```python
from build123d import *

# Parameters (mm, degrees)
BOSS_EXTRU_1_DEPTH = 3


with BuildPart() as part:
    # Esquisse1 → Boss.-Extru.1 (new body)
    with BuildSketch(Plane.XY):
        Polygon((-113.35310374, -10.173637327), (-129.143746737, -14.701531345), (-206.446773007, -14.701531345), (-222.237416003, -10.173637327), (-228.962816583, -8.245159743), (-248.413999189, -2.668793647), (-249.872259625, -3.248768002), (-288.323340616, 7.774587685), (-289.252816682, 9.039090747), (-323.901077775, 18.972234266), (-327.912092601, 16.748746626), (-350.173506381, -60.88602933), (-347.950273, -64.896848521), (-291.80662177, -80.995781451), (-285.908889082, -97.08692424), (-249.107067355, -113.823629959), (-232.032352152, -131.457901649), (-227.449883961, -131.529994355), (-199.380152195, -104.350948678), (-136.210367548, -104.350948678), (-108.140635782, -131.529994355), (-103.558167591, -131.457901649), (-86.483452388, -113.823629959), (-49.681630661, -97.08692424), (-43.783897973, -80.995781451), (12.359753257, -64.896848521), (14.582986638, -60.88602933), (-7.678427142, 16.748746626), (-11.689441968, 18.972234266), (-46.337703061, 9.039090747), (-47.267179127, 7.774587685), (-85.718260118, -3.248768002), (-87.176520554, -2.668793647), (-106.62770316, -8.245159743), align=None)
        Polygon((-210.232188047, -30.001147656), (-224.390430785, -79.377961929), (-208.212806214, -96.161100182), (-207.491865187, -96.85509979), (-208.236606037, -97.572971364), (-229.533063287, -118.225792128), (-242.655085998, -104.673746846), (-258.969310369, -95.012679745), (-277.629290011, -88.825419148), (-272.289144354, -70.202118055), (-298.538981418, -62.6750984), (-299.849714513, -67.246167925), (-337.461409717, -56.461187875), (-321.404434006, -0.463858857), (-284.873898651, -10.938821309), (-283.564528345, -6.372504389), (-265.299260667, -11.609985616), (-264.679553884, -9.448811229), (-245.452786066, -14.960840928), (-246.072799476, -17.123084647), (-227.807531798, -22.360565873), (-228.496674065, -24.763890567), align=None, mode=Mode.SUBTRACT)
        Polygon((-106.057456456, -118.225792128), (-128.0696158, -96.878899722), (-127.377713529, -96.161100182), (-111.200088958, -79.377961929), (-125.358331696, -30.001147656), (-107.093845678, -24.763890567), (-107.782987945, -22.360565873), (-89.517720268, -17.123084647), (-90.137733677, -14.960840928), (-70.910965859, -9.448811229), (-70.291259076, -11.609985616), (-52.025991399, -6.372504389), (-50.716621092, -10.938821309), (-14.186085737, -0.463858857), (1.870889973, -56.461187875), (-35.740805231, -67.246167925), (-37.051538325, -62.6750984), (-63.301375389, -70.202118055), (-57.961229733, -88.825419148), (-76.621209374, -95.012679745), (-92.935433745, -104.673746846), align=None, mode=Mode.SUBTRACT)
    extrude(amount=BOSS_EXTRU_1_DEPTH)


solid = part.part
```
CAD build for the part. Positions are in the model's coordinates, mm. A direction names the side the tool comes from. Round coordinates to 2 decimals unless told otherwise and drop trailing zeros. Order: outer loops, then holes, each group sorted by start corner. A loop starts at its lowest first (then second) coordinate and runs counter-clockwise, first axis right, second up. Notation, with made-up numbers: (-20.5, 70.5) - (38.5, 70.5) arc R15 ccw to (38.5, 79.5) - close; hole circle Ø1 at (35.5, -19.75). An arc over 180 degrees is marked (long way). Answer as CSV lines item,"result". Start each with the question number.
1. Pin check, flat tips, straight feed: pin 1 (10 mm diameter, centred on x = -309, y = -85, fed in from -Z); pin 2 (1.5 mm diameter, centred on x = -168, z = 1, fed in from -Y); pin 3 (1 mm diameter, centred on x = -184.5, z = 1, fed in from +Y). Stop position of each tip, or through.
2. Drill centre lines: L1, parallel to X at y = -55, z = 1.4; L2, parallel to X at y = -33, z = 2.15; L3, parallel to X at y = -107, z = 1.1. Where is each one in solid material? Low to high. Write a range as [from, to].
3. Saw through at A-A, the plane x = -304. Write the cut outline in (y, z), and give its area (3 significant figures).
4. Saw through at B-B, the plane y = -44. Write the cut outline in (x, z), and give its area (3 significant figures).
5. Saw through at D-D, the plane x = -144.5. Write the cut outline in (y, z).
6. Pull direction X, two halves, no side cores. Call faces 4 (the face through (-68.34, -105.572, 1.479)), 5 (the face through (-170, -55, 0)), 6 (the face through (-218.736, -107.755, 1.479)): +X half, -X half, draft (parallel to the pull), parting line (faces both ways), or undercut.
7. Saw through at C-C, the plane z = 1.9. Count the separate pieces of the cut face and the enclosed holes in it, and give its area (3 significant figures).
8. Tool access for faces 1 (the face through (-122.37, -117.75, 1.48)), 2 (the face through (-306.334, 13.936, 1.479)), 3 (the face through (-268.17, -91.96, 1.48)): list every direction of +Z, -Z, +X, -X, +Y, -Y with a clear straight run to the whole face (end or side of a thin tool).
Model answer:
1,pin 1,"passes through"
1,pin 2,"stops at y = -104.35"
1,pin 3,"stops at y = -14.7"
2,L1,"x = [-348.49, -337.04], [-217.4, -118.19], [1.45, 12.9]"
2,L2,"x = [-342.18, -330.73], [-211.09, -124.5], [-4.86, 6.59]"
2,L3,"x = [-264.11, -240.4], [-217.96, -202.12], [-133.47, -117.63], [-95.19, -71.48]"
3,outline,"(-77.5, 0) - (-66.06, 0) - (-66.06, 3) - (-77.5, 3) - close; (-5.45, 0) - (13.27, 0) - (13.27, 3) - (-5.45, 3) - close"
3,area,"90.5 mm²"
4,outline,"(-345.33, 0) - (-333.89, 0) - (-333.89, 3) - (-345.33, 3) - close; (-214.25, 0) - (-121.34, 0) - (-121.34, 3) - (-214.25, 3) - close; (-1.7, 0) - (9.74, 0) - (9.74, 3) - (-1.7, 3) - close"
4,area,"347 mm²"
5,outline,"(-104.35, 0) - (-14.7, 0) - (-14.7, 3) - (-104.35, 3) - close"
6,face 4,"+X half"
6,face 5,"draft"
6,face 6,"undercut"
7,separate pieces,"1"
7,enclosed holes,"2"
7,area,"17,800 mm²"
8,face 1,"+Z, -Z, -Y"
8,face 2,"+Z, -Z, +Y"
8,face 3,"+Z, -Z"
